Job drawing, mm, ordinate dimensions from the low corner. One solid piece. A direction names the side the tool comes from. Give positions to 0.01 mm unless a question says otherwise; leave off trailing zeros. Order: outer loops, then holes, each group sorted by start corner. A loop starts at its lowest first (then second) coordinate and runs counter-clockwise, first axis right, second up.
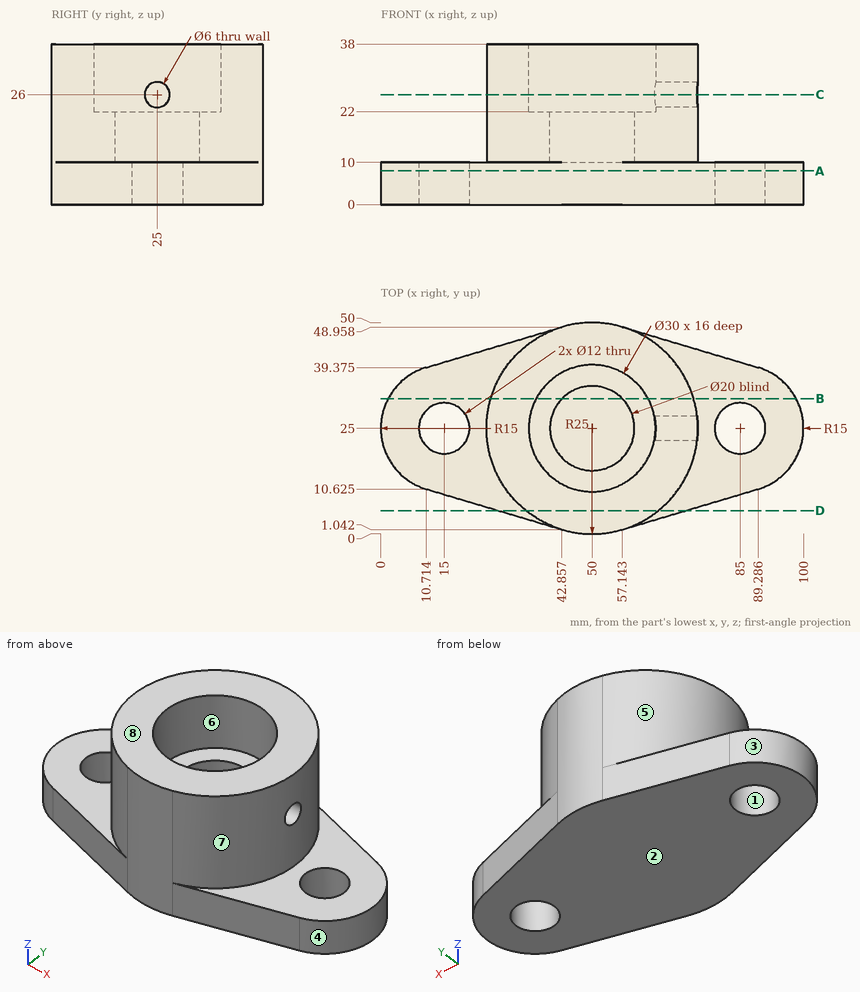
Item 1: Band-saw the part on B-B on y = 32. List the corners of the cut face in (x, z).
Item 2: Drop flat-ended pins along their axis: P1, Ø3, axis at y = 42, z = 19.5, coming from the +X side (1 decimal); P2, Ø16, axis at x = 45.5, y = 26, coming from the +Z side; P3, Ø6, axis at y = 7, z = 27, coming from the -X side; P4, Ø16, axis at x = 50, y = 25, coming from the -Z side. Give the stop position or say it passes through.
Item 3: Drill centre lines: probe 1 along Y at (x, z) = (50, 27); probe 2 along Z at (x, y) = (10.5, 17); probe 3 along Y at (x, z) = (41, 27) (1 decimal). Where is each one in solid material? Low to high.
Item 4: Band-saw the part on D-D on y = 5.5. List the corners of the cut face in (x, z) (1 decimal), plus the area to 3 significant figures.
Item 5: Which spindle directions (+Z, -Z, +X, -X, +Y, -Y) get a long thin tool onto all of the face, cutting with end or side? Do the marked faces 4, 5, 6, 7 and 8. Say none if no direction does.
Item 6: Band-saw the part on C-C on z = 26. List the corners of the cut face in (x, y), plus the area to 3 significant figures.
Item 7: Band-saw the part on A-A on z = 8. List the corners of the cut face in (x, y) (1 decimal).
Item 8: Pull direction X, two halves, no side cores. Call the marked faces 1, 2 and 3: released by +X, released by -X, zero draft, split by the parting line, or undercut.
Working result:
1. outline: (1.73, 0) - (98.27, 0) - (98.27, 10) - (74, 10) - (74, 38) - (63.27, 38) - (63.27, 22) - (57.14, 22) - (57.14, 10) - (42.86, 10) - (42.86, 22) - (36.73, 22) - (36.73, 38) - (26, 38) - (26, 10) - (1.73, 10) - close
2. P1: stops at x = 69.6
2. P2: stops at z = 22
2. P3: stops at x = 30
2. P4: stops at z = 0
3. probe 1: y = 0 to 10, 40 to 50
3. probe 2: z = 0 to 10
3. probe 3: y = 1.7 to 13, 37 to 48.3
4. outline: (27.9, 0) - (72.1, 0) - (72.1, 10) - (65.6, 10) - (65.6, 38) - (34.4, 38) - (34.4, 10) - (27.9, 10) - close
4. area: 1,320 mm2
5. face 4: +Z, -Z, +X
5. face 5: +Z, -X
5. face 6: +Z
5. face 7: +Z, +X
5. face 8: +Z, +X, -X, +Y, -Y
6. outline: (57.14, 48.96) arc R25 ccw (long way) to (74.82, 22) - (64.7, 22) arc R15 cw (long way) to (64.7, 28) - (74.82, 28) arc R25 ccw to start
6. area: 1,200 mm2
7. outline: (10.7, 10.6) - (42.9, 1) arc R25 ccw to (57.1, 1) - (89.3, 10.6) arc R15 ccw to (89.3, 39.4) - (57.1, 49) arc R25 ccw to (42.9, 49) - (10.7, 39.4) arc R15 ccw to start; hole circle Ø12 at (15, 25); hole circle Ø12 at (85, 25)
8. face 1: undercut
8. face 2: zero draft
8. face 3: released by -X
